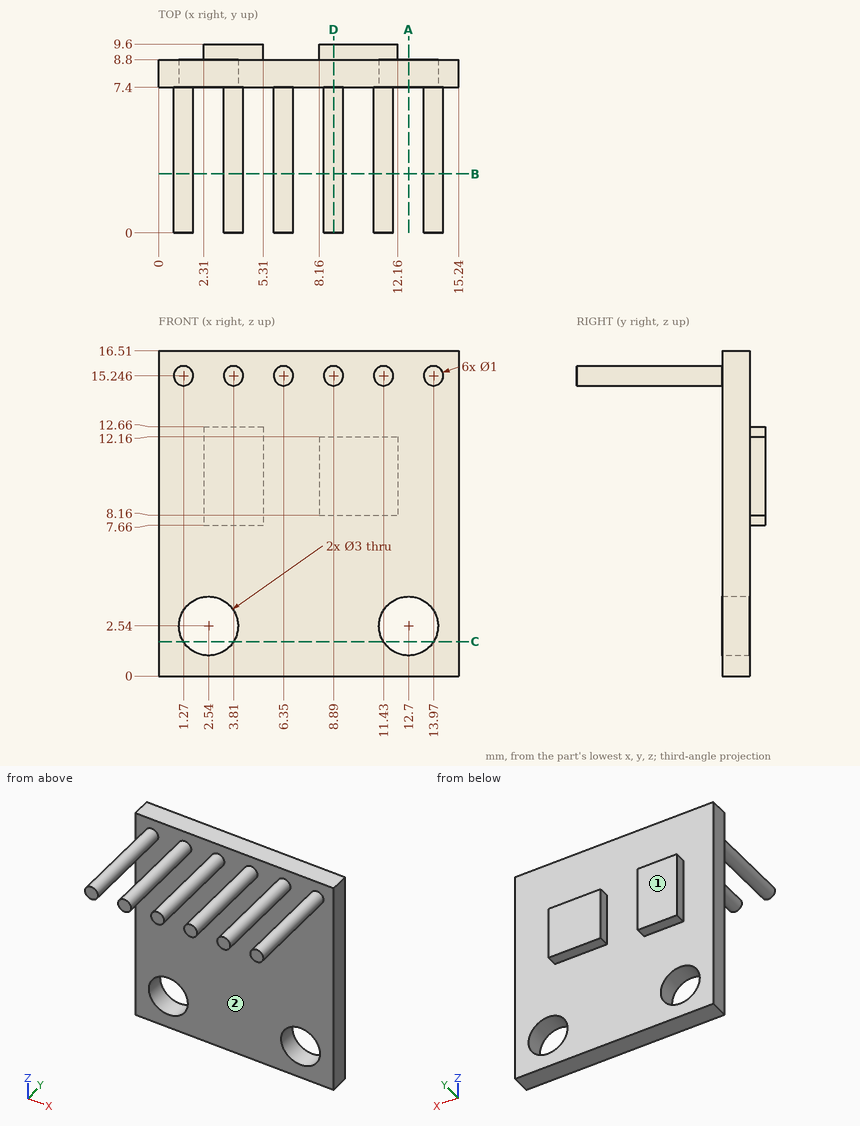
Verification items for this drawing (mm, ordinates from the low corner). Coordinates: 2 decimals unless noted, no trailing zeros. Order: outer loops, then holes, each group sorted by start corner. A loop starts at its lowest first (then second) coordinate and runs counter-clockwise, first axis right, second up. Notation, with made-up numbers: (16.25, 65) - (28.25, 65) arc R17 ccw to (28.25, 96) - close; hole circle Ø10 at (-34.5, 19). An arc over 180 degrees is marked (long way). Answer in a Markdown table with one row per item. Add a question column.
1. Section check A-A (x = 12.7). Enter the section's corners in (y, z).
2. Section check B-B (y = 3). Enter the section's corners in (x, z).
3. Section check D-D (x = 8.89). Enter the section's corners in (y, z), plus the area to 3 significant figures.
4. Material ranges on L1, parallel to X at y = 8.05, z = 2.54; L2, parallel to Y at x = 9.5, z = 11.5; L3, parallel to Y at x = 7.25, z = 2.25, recorded low to high. Write a range as [from, to].
5. Draft check along Y on the marked faces 1 and 2. Enter one of: +Y half, -Y half, draft (parallel to the pull), parting line (faces both ways), or undercut.
6. Gauge pin test, flat ends, axial feed: pin 1 Ø5 at (x, z) = (2.54, 2.54) entering from -Y; pin 2 Ø2 at (x, y) = (11.5, 3) entering from -Z; pin 3 Ø0.9 at (y, z) = (9.5, 10) entering from -X. Record the tip position at first contact, or that the pin passes through.
7. Section check C-C (z = 1.75). Enter the section's corners in (x, y) (3 decimals), plus the area to 3 significant figures.
Data:
| question | item | result |
|---|---|---|
| 1 | outline | (7.4, 0) - (8.8, 0) - (8.8, 1.04) - (7.4, 1.04) - close; (7.4, 4.04) - (8.8, 4.04) - (8.8, 16.51) - (7.4, 16.51) - close |
| 2 | outline | circle Ø1 at (1.27, 15.25); circle Ø1 at (3.81, 15.25); circle Ø1 at (6.35, 15.25); circle Ø1 at (8.89, 15.25); circle Ø1 at (11.43, 15.25); circle Ø1 at (13.97, 15.25) |
| 3 | outline | (0, 14.75) - (7.4, 14.75) - (7.4, 0) - (8.8, 0) - (8.8, 8.16) - (9.6, 8.16) - (9.6, 12.16) - (8.8, 12.16) - (8.8, 16.51) - (7.4, 16.51) - (7.4, 15.75) - (0, 15.75) - close |
| 3 | area | 33.7 mm² |
| 4 | L1 | x = [0, 1.04], [4.04, 11.2], [14.2, 15.24] |
| 4 | L2 | y = [7.4, 9.6] |
| 4 | L3 | y = [7.4, 8.8] |
| 5 | face 1 | +Y half |
| 5 | face 2 | -Y half |
| 6 | pin 1 | stops at y = 7.4 |
| 6 | pin 2 | stops at z = 14.75 |
| 6 | pin 3 | stops at x = 2.31 |
| 7 | outline | (0, 7.4) - (1.265, 7.4) - (1.265, 8.8) - (0, 8.8) - close; (3.815, 7.4) - (11.425, 7.4) - (11.425, 8.8) - (3.815, 8.8) - close; (13.975, 7.4) - (15.24, 7.4) - (15.24, 8.8) - (13.975, 8.8) - close |
| 7 | area | 14.2 mm² |
